Autodesk Inventor part; units mm, degrees
ref_plane "YZ Plane" through (0, 0, 0) normal (1, 0, 0) x (0, 1, 0)
ref_plane "XZ Plane" through (0, 0, 0) normal (0, 1, 0) x (-1, 0, 0)
ref_plane "XY Plane" through (0, 0, 0) normal (0, 0, 1) x (1, 0, 0)
sketch "Sketch1" plane through (0, 0, 0) normal (0, 1, 0) x (-1, 0, 0)
  circle A0 centre (0, 0) radius 9.525
  line L0 (6.3918, 3.5928) -> (6.3073, -3.7391)
  line L1 (6.3073, -3.7391) -> (-0.0845, -7.3319)
  line L2 (-0.0845, -7.3319) -> (-6.3918, -3.5928)
  line L3 (-6.3918, -3.5928) -> (-6.3073, 3.7391)
  line L4 (-6.3073, 3.7391) -> (0.0845, 7.3319)
  line L5 (0.0845, 7.3319) -> (6.3918, 3.5928)
  point P0 (6.3496, -0.0731)
  dimension "d0" = 19.05
  dimension "d1" = 12.7
extrude "Extrusion1" add sketch "Sketch1" along normal blind 6.35
properties part number "spacer"
Geometry check sheet. Reference: the model listing, model coordinates, mm. A direction names the side the tool comes from. Round coordinates to 2 decimals unless told otherwise and drop trailing zeros. Loops run counter-clockwise (first coordinate to the right, second up) from the corner with the lowest first, then second, coordinate; pieces in that order, holes last. Notation, with made-up numbers: (60.5, 42) - (101.5, 42) arc R25 ccw to (101.5, 73) - close; hole circle Ø6 at (76, 20.5). An arc over 180 degrees is marked (long way). Use a Markdown table: item, result.
Q1. Cross-section at A-A on z = -3. Record the cut outline in (x, y).
Solutions:
| item | result |
|---|---|
| outline | (-9.04, 0) - (-6.32, 0) - (-6.32, 6.35) - (-9.04, 6.35) - close; (6.38, 0) - (9.04, 0) - (9.04, 6.35) - (6.38, 6.35) - close |
Q2. Draft check along Z on faces 3 (the cylindrical face through (7.559, 3.131, 5.796)), 4 (the flat face through (-3.19, 3.13, 5.49)), 5 (the flat face through (2.3, 0, -6.2)). Enter one of: released by +Z, released by -Z, zero draft, split by the parting line, or undercut.
Solutions:
| item | result |
|---|---|
| face 3 | split by the parting line |
| face 4 | undercut |
| face 5 | zero draft |
Q3. Go/stop test with flat-tipped pins: P1, Ø1, axis at x = -4.5, y = 2, coming from the +Z side; P2, Ø1, axis at y = 5, z = 6.5, coming from the -X side; P3, Ø1.5, axis at x = 7, y = 3, coming from the -Z side; P4, Ø3, axis at x = 0, z = 3.5, coming from the -Y side. Record where each tip stops, or that it passes through.
Solutions:
| item | result |
|---|---|
| P1 | stops at z = 8.64 |
| P2 | stops at x = -7.4 |
| P3 | stops at z = -7.19 |
| P4 | passes through |
Q4. Cross-section at B-B on x = -6. Record the cut outline in (y, z), plus the area to 3 significant figures.
Solutions:
| item | result |
|---|---|
| outline | (0, -7.4) - (6.35, -7.4) - (6.35, -3.91) - (0, -3.91) - close; (0, 3.83) - (6.35, 3.83) - (6.35, 7.4) - (0, 7.4) - close |
| area | 44.8 mm2 |
Q5. Material ranges on line 1 (Z direction, x = -0.5, y = 1.25); line 2 (X direction, y = 6.25, z = 2.5); line 3 (Z direction, x = -3.5, y = 3.75), recorded low to high.
Solutions:
| item | result |
|---|---|
| line 1 | z = -9.51 to -7, 7.09 to 9.51 |
| line 2 | x = -9.19 to -6.38, 6.32 to 9.19 |
| line 3 | z = -8.86 to -5.32, 5.31 to 8.86 |
Q6. Access from +Z, -Z, +X, -X, +Y, -Y to the whole of each face (thin tool, end or side, straight path). Record for faces 1 (the flat face through (3.19, 3.13, -5.49)), 2 (the flat face through (2.3, 6.35, -6.2)).
Solutions:
| item | result |
|---|---|
| face 1 | +Y, -Y |
| face 2 | +Z, -Z, +X, -X, +Y |
